```python
from build123d import *

# Parameters (mm, degrees)
F1_DEPTH = 10
F3_DEPTH = 75
F5_DEPTH = 25


with BuildPart() as f1:
    # F0 (on Top) → F1 (new body)
    with BuildSketch(Plane.XY):
        with BuildLine():
            ThreePointArc((237.5, 0), (0, -237.5), (-237.5, 0))
            Line((-237.5, 0), (-237.5, 500))
            Line((-237.5, 500), (-275, 500))
            Line((-275, 500), (-275, -500))
            Line((-275, -500), (275, -500))
            Line((275, -500), (275, 500))
            Line((275, 500), (237.5, 500))
            Line((237.5, 500), (237.5, 0))
        make_face()
    extrude(amount=F1_DEPTH)

    # F2 (on face) → F3 (join)
    with BuildSketch(Plane(origin=(0, 0, 0), x_dir=(1, 0, 0), z_dir=(0, 0, -1))):
        with BuildLine():
            Line((-237.5, 500), (-237.5, 0))
            ThreePointArc((-237.5, 0), (0, 237.5), (237.5, 0))
            Line((237.5, 0), (237.5, 500))
            Line((237.5, 500), (-237.5, 500))
        make_face()
    extrude(amount=F3_DEPTH)

    # F4 (on face) → F5 (join)
    with BuildSketch(Plane(origin=(0, 0, -75), x_dir=(1, 0, 0), z_dir=(0, 0, -1))):
        with BuildLine():
            ThreePointArc((70.887234, 500), (156.568516, 480.115923), (237.5, 445.666636))
            Line((237.5, 445.666636), (237.5, 456.966903))
            ThreePointArc((237.5, 456.966903), (181.723121, 481.873124), (123.389627, 500))
            Line((123.389627, 500), (70.887234, 500))
        make_face()
        with BuildLine():
            ThreePointArc((-123.389627, 500), (-181.723121, 481.873124), (-237.5, 456.966903))
            Line((-237.5, 456.966903), (-237.5, 445.666636))
            ThreePointArc((-237.5, 445.666636), (-156.568516, 480.115923), (-70.887234, 500))
            Line((-70.887234, 500), (-123.389627, 500))
        make_face()
    extrude(amount=F5_DEPTH)


solid = f1.part
```
Geometry check sheet. Reference: the model listing, model coordinates, mm. A direction names the side the tool comes from. Give positions to 0.01 mm unless a question says otherwise; leave off trailing zeros. Order: outer loops, then holes, each group sorted by start corner. A loop starts at its lowest first (then second) coordinate and runs counter-clockwise, first axis right, second up.
1. Section check A-A, the plane z = -84.5. Enter the section's corners in (x, y).
2. Gauge pin test, flat ends, axial feed: pin 1 Ø21.5 at (x, y) = (-162.5, -468) entering from -Z; pin 2 Ø19 at (x, y) = (-254, 49.5) entering from -Z; pin 3 Ø1.5 at (x, z) = (-81.5, -76) entering from +Y; pin 4 Ø2 at (y, z) = (-386, -73.5) entering from +X. Record the tip position at first contact, or that the pin passes through.
3. Access from +Z, -Z, +X, -X, +Y, -Y to the whole of each face (thin tool, end or side, straight path). Record for faces 4 (the face through (-257, 7, 0)), 5 (the face through (-207, -488, -75)), 6 (the face through (-157.74, -479.732, -87.325)).
4. Section check B-B, the plane y = 176. Enter the section's corners in (x, z), and give its area (3 significant figures).
5. Thickness scan on L1, parallel to X at y = 70.5, z = 4; L2, parallel to Z at x = -14, y = -458.5; L3, parallel to X at y = -42, z = -20.5. Record the ranges inside material, lowest first.
6. Section check C-C, the plane y = -309. Enter the section's corners in (x, z), and give its area (3 significant figures).
7. Section check D-D, the plane x = 0. Enter the section's corners in (y, z), and give its area (3 significant figures).
8. Release check for a two-part mould opening along X. For faces 1 (the face through (-237.5, -253, -38)), 2 (the face through (-3, -365, -75)), 3 (the face through (4, -500, -32)) record: pulls with the +X half, pulls with the -X half, needs draft (parallel to the pull), parting line crosses it, or undercut.
Values follow:
1. outline: (-237.5, -456.97) arc R515 ccw to (-123.39, -500) - (-70.89, -500) arc R505 cw to (-237.5, -445.67) - close; (70.89, -500) - (123.39, -500) arc R515 ccw to (237.5, -456.97) - (237.5, -445.67) arc R505 cw to start
2. pin 1: stops at z = -100
2. pin 2: stops at z = 0
2. pin 3: stops at y = -498.26
2. pin 4: stops at x = 237.5
3. face 4: -Z, -X, +Y, -Y
3. face 5: -Z, -X, -Y
3. face 6: -Z, +Y
4. outline: (-275, 0) - (-237.5, 0) - (-237.5, 10) - (-275, 10) - close; (237.5, 0) - (275, 0) - (275, 10) - (237.5, 10) - close
4. area: 750 mm2
5. L1: x = -275 to -237.5, 237.5 to 275
5. L2: z = -75 to 10
5. L3: x = -237.5 to -233.76, 233.76 to 237.5
6. outline: (-275, 0) - (-237.5, 0) - (-237.5, -75) - (237.5, -75) - (237.5, 0) - (275, 0) - (275, 10) - (-275, 10) - close
6. area: 41,100 mm2
7. outline: (-500, -75) - (-237.5, -75) - (-237.5, 10) - (-500, 10) - close
7. area: 22,300 mm2
8. face 1: pulls with the -X half
8. face 2: undercut
8. face 3: needs draft
